Source: CAD feature listing. Evaluate the final solid. Frame: model axes, mm. Round coordinates to 2 decimals unless told otherwise and drop trailing zeros. Loops run counter-clockwise (first coordinate to the right, second up) from the corner with the lowest first, then second, coordinate; pieces in that order, holes last.
Item 1: Section query C-C on y = 2.5. Return loops of the section in (x, z) (3 decimals), then the cut area to 3 significant figures.
Item 2: Section query D-D on x = 201.5. Return loops of the section in (y, z).
Item 3: Section query B-B on z = 26. Return loops of the section in (x, y).
Item 4: Ray query, L1, parallel to Z at x = 273.3, y = 3; L2, parallel to Z at x = 71, y = 5.5; L3, parallel to X at y = 2.25, z = -58. Return the intervals inside material, ascending.
Item 5: Section query A-A on x = 273.3. Return loops of the section in (y, z), then the cut area to 3 significant figures.
```python
from build123d import *

# Parameters (mm, degrees)
SKETCH1_W           = 286.791999948
SKETCH1_H           = 286.791999948
BOSS_EXTRUDE1_DEPTH = 6.35
SKETCH2_R           = 10
SKETCH2_W           = 180.979932016
SKETCH2_H           = 187.647432016
CUT_EXTRUDE1_DEPTH  = 6.35
FILLET1_R           = 3.175


with BuildPart() as part:
    # Sketch1 → Boss-Extrude1 (new body)
    with BuildSketch(Plane(origin=(0, 0, 0), x_dir=(1, 0, 0), z_dir=(0, 1, 0))):
        with Locations((143.395999974, 0)):
            Rectangle(SKETCH1_W, SKETCH1_H)
    extrude(amount=BOSS_EXTRUDE1_DEPTH)

    # Sketch2 → Cut-Extrude1 (cut)
    with BuildSketch(Plane.XZ):
        with Locations(Location((273.299999948, -129.903999974, 0), (0, 0, 270))):
            Circle(SKETCH2_R)
        with Locations(Location((14, -129.903999974, 0), (0, 0, 270))):
            Circle(SKETCH2_R)
        with Locations(Location((14, 129.395999974, 0), (0, 0, 270))):
            Circle(SKETCH2_R)
        with Locations(Location((273.299999948, 129.395999974, 0), (0, 0, 270))):
            Circle(SKETCH2_R)
        with Locations((143.649999974, -0.254)):
            Rectangle(SKETCH2_W, SKETCH2_H)
    extrude(amount=-CUT_EXTRUDE1_DEPTH, mode=Mode.SUBTRACT)

    # Fillet1
    fillet1_edges = [part.edges().sort_by_distance(p)[0] for p in [
        (53.160033966, 3.175, -94.077716008),
        (53.160033966, 3.175, 93.569716008),
        (234.139965982, 3.175, 93.569716008),
        (234.139965982, 3.175, -94.077716008),
    ]]
    fillet(fillet1_edges, radius=FILLET1_R)


solid = part.part
```
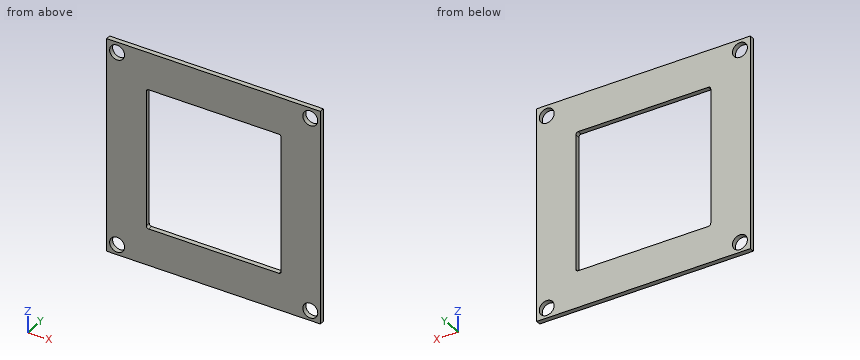
Data:
1. outline: (0, -143.396) - (286.792, -143.396) - (286.792, 143.396) - (0, 143.396) - close; hole circle Ø20 at (14, -129.904); hole circle Ø20 at (14, 129.396); hole (53.16, -90.903) arc R3.175 ccw to (56.335, -94.078) - (230.965, -94.078) arc R3.175 ccw to (234.14, -90.903) - (234.14, 90.395) arc R3.175 ccw to (230.965, 93.57) - (56.335, 93.57) arc R3.175 ccw to (53.16, 90.395) - close; hole circle Ø20 at (273.3, -129.904); hole circle Ø20 at (273.3, 129.396)
1. area: 47,000 mm2
2. outline: (0, -143.4) - (6.35, -143.4) - (6.35, -94.08) - (0, -94.08) - close; (0, 93.57) - (6.35, 93.57) - (6.35, 143.4) - (0, 143.4) - close
3. outline: (0, 0) - (53.16, 0) - (53.16, 6.35) - (0, 6.35) - close; (234.14, 0) - (286.79, 0) - (286.79, 6.35) - (234.14, 6.35) - close
4. L1: z = -143.4 to -139.9, -119.9 to 119.4, 139.4 to 143.4
4. L2: z = -143.4 to -94.08, 93.57 to 143.4
4. L3: x = 0 to 53.16, 234.14 to 286.79
5. outline: (0, -143.4) - (6.35, -143.4) - (6.35, -139.9) - (0, -139.9) - close; (0, -119.9) - (6.35, -119.9) - (6.35, 119.4) - (0, 119.4) - close; (0, 139.4) - (6.35, 139.4) - (6.35, 143.4) - (0, 143.4) - close
5. area: 1,570 mm2
